Read the model definition and answer for the solid it produces. Units are mm, in the model's axes. Face numbers are marked on the shaded views. A direction names the side the tool comes from. Give positions to 0.01 mm unless a question says otherwise; leave off trailing zeros. Write each loop counter-clockwise with the first axis right and the second up, starting at its lowest first coordinate (ties: lowest second). Pieces come first, ordered by that corner, then holes. Notation, with made-up numbers: (-23, 9.5) -> (-6, 9.5) arc R31 ccw to (-6, 41.5) -> close; hole circle Ø6 at (53, -19). An arc over 180 degrees is marked (long way). Answer as CSV lines item,"result". Start each with the question number.
1. The part is cut by section C-C, the plane y = 531.5. Determine the outline of the cut face in (x, z).
2. Given pin 1 (7.5 mm diameter, centred on x = 5.715, z = 291.592, fed in from -Y); pin 2 (5 mm diameter, centred on x = 15.24, y = 520.7, fed in from -Z); pin 3 (3 mm diameter, centred on y = 525, z = 280, fed in from +X), each flat-ended and moving along its own axis, determine where each tip first touches the part or whether it passes through.
3. Find the intervals of material crossed by line 1 (Z direction, x = 22, y = 526); line 2 (Y direction, x = 15.24, z = 303.95); line 3 (Y direction, x = 28, z = 278.75), in increasing order.
4. The part is cut by section B-B, the plane y = 520.7. Determine the outline of the cut face in (x, z), and give its area (3 significant figures).
5. A tool of negligible diameter and unlimited length cuts with its end or side. For the marked faces 5 and 6, from which of +Z, -Z, +X, -X, +Y, -Y can it reach the whole face along a straight path? Write none if from no direction.
6. For a pull along Z with two mould halves and no side action, classify the marked faces 1, 2, 3 and 4 as pulls with the +Z half, pulls with the -Z half, needs draft (parallel to the pull), parting line crosses it, or undercut.
7. The part is cut by section A-A, the plane x = 15.24. Give the number of separate pieces and of enclosed holes in the cut face, and give its area (3 significant figures).
8. The part is cut by section D-D, the plane x = 24. Determine the outline of the cut face in (y, z) (1 decimal).
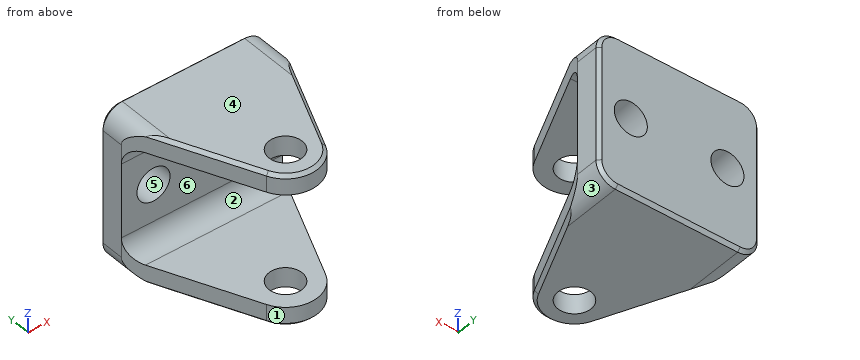
from build123d import *

# Parameters (mm, degrees)
BULK_TRIANGLE_DEPTH      = 14.9225
BULK_TRIANGLE_DEPTH_BACK = 14.9225
U_CUTOUT_DEPTH           = 627.44103
U_CUTOUT_DEPTH_BACK      = 627.44103
F_1_4_CLEARANCE_HOLE1_D  = 6.5278
F_1_4_CLEARANCE_HOLE2_D  = 6.5278
INNER_FILLET_R           = 3.81
TRIANGLE_DEBURR_SIZE     = 0.635
OUTER_FILLET_R           = 3.81
CLAMP_FACE_DEBURR_SIZE   = 0.635


with BuildPart() as part:
    # Sketch1 → Bulk Triangle (new, two sides)
    with BuildSketch(Plane.XY.offset(291.592)) as bulk_triangle_sk:
        with BuildLine():
            Line((9.42744, 518.143313), (-0.635, 541.02))
            Line((-0.635, 541.02), (-0.635, 546.1))
            Line((-0.635, 546.1), (31.115, 546.1))
            Line((31.115, 546.1), (31.115, 541.02))
            Line((31.115, 541.02), (21.05256, 518.143313))
            ThreePointArc((21.05256, 518.143313), (15.24, 514.35), (9.42744, 518.143313))
        make_face()
    extrude(amount=BULK_TRIANGLE_DEPTH)
    extrude(bulk_triangle_sk.sketch, amount=-BULK_TRIANGLE_DEPTH_BACK)

    # Sketch3 → U-Cutout (cut, two sides)
    with BuildSketch(Plane(origin=(15.24, 0, 0), x_dir=(0, -4.31797119152115e-05, -0.9999999990677564), z_dir=(1, 0, 0))) as u_cutout_sk:
        Polygon((-302.727861, 541.006929), (-302.726709, 514.336929), (-280.501709, 514.337888), (-280.502861, 541.007888), align=None)
    extrude(amount=U_CUTOUT_DEPTH, mode=Mode.SUBTRACT)
    extrude(u_cutout_sk.sketch, amount=-U_CUTOUT_DEPTH_BACK, mode=Mode.SUBTRACT)

    # 1/4 Clearance Hole1 (through all)
    with Locations(Plane(origin=(15.24, 520.7, 306.5145), x_dir=(1, 0, 0), z_dir=(0, 0, 1))):
        with Locations((0, 0)):
            Hole(F_1_4_CLEARANCE_HOLE1_D / 2)

    # 1/4 Clearance Hole2 (through all)
    with Locations(Plane(origin=(24.765, 541.02, 291.592), x_dir=(-1, 0, 0), z_dir=(0, -1, 0))):
        with Locations((0, 0), (19.05, 0)):
            Hole(F_1_4_CLEARANCE_HOLE2_D / 2)

    # Inner Fillet
    inner_fillet_edges = [part.edges().sort_by_distance(p)[0] for p in [
        (15.24, 541.02, 280.4795),
        (15.24, 541.02, 302.7045),
    ]]
    fillet(inner_fillet_edges, radius=INNER_FILLET_R)

    # Triangle Deburr
    triangle_deburr_edges = [part.edges().sort_by_distance(p)[0] for p in [
        (15.24, 514.35, 276.6695),
        (4.39622, 529.581656, 276.6695),
        (26.08378, 529.581656, 276.6695),
        (4.39622, 529.581656, 306.5145),
        (15.24, 514.35, 306.5145),
        (26.08378, 529.581656, 306.5145),
    ]]
    chamfer(triangle_deburr_edges, length=TRIANGLE_DEBURR_SIZE)

    # Outer Fillet
    outer_fillet_edges = [part.edges().sort_by_distance(p)[0] for p in [
        (-0.635, 544.348569, 276.6695),
        (31.115, 544.348569, 276.6695),
        (-0.635, 544.348569, 306.5145),
        (31.115, 544.348569, 306.5145),
    ]]
    fillet(outer_fillet_edges, radius=OUTER_FILLET_R)

    # Clamp Face Deburr
    clamp_face_deburr_edges = [part.edges().sort_by_distance(p)[0] for p in [
        (-0.635, 546.1, 291.592),
        (15.24, 546.1, 276.6695),
        (31.115, 546.1, 291.592),
        (15.24, 546.1, 306.5145),
        (29.999077, 546.1, 305.398577),
        (0.480923, 546.1, 305.398577),
        (29.999077, 546.1, 277.785423),
        (0.480923, 546.1, 277.785423),
    ]]
    chamfer(clamp_face_deburr_edges, length=CLAMP_FACE_DEBURR_SIZE)


solid = part.part
Results found:
1,outline,"(3.55, 277.3) -> (4.25, 276.67) -> (26.23, 276.67) -> (26.93, 277.3) -> (26.93, 280.48) -> (3.55, 280.48) -> close; (3.55, 302.7) -> (26.93, 302.7) -> (26.93, 305.88) -> (26.23, 306.51) -> (4.25, 306.51) -> (3.55, 305.88) -> close"
2,pin 1,"stops at y = 541.02"
2,pin 2,"passes through"
2,pin 3,"stops at x = 24.73"
3,line 1,"z = 276.67 to 280.48, 302.7 to 306.51"
3,line 2,"y = 514.35 to 517.44, 523.96 to 546.1"
3,line 3,"y = 533.94 to 546.1"
4,outline,"(8.3, 277.3) -> (9, 276.67) -> (11.98, 276.67) -> (11.98, 280.48) -> (8.3, 280.48) -> close; (8.3, 302.7) -> (11.98, 302.7) -> (11.98, 306.51) -> (9, 306.51) -> (8.3, 305.88) -> close; (18.5, 276.67) -> (21.48, 276.67) -> (22.18, 277.3) -> (22.18, 280.48) -> (18.5, 280.48) -> close; (18.5, 302.7) -> (22.18, 302.7) -> (22.18, 305.88) -> (21.48, 306.51) -> (18.5, 306.51) -> close"
4,area,"55.1 mm²"
5,face 5,"+Y, -Y"
5,face 6,"+X, -X, -Y"
6,face 1,"needs draft"
6,face 2,"undercut"
6,face 3,"pulls with the -Z half"
6,face 4,"pulls with the +Z half"
7,separate pieces,"3"
7,enclosed holes,"0"
7,area,"311 mm²"
8,outline,"(524.8, 277.3) -> (526.4, 276.7) -> (545.5, 276.7) -> (546.1, 277.3) -> (546.1, 288.4) -> (541, 288.4) -> (541, 284.3) arc R3.8 cw to (537.2, 280.5) -> (524.8, 280.5) -> close; (524.8, 302.7) -> (537.2, 302.7) arc R3.8 cw to (541, 298.9) -> (541, 294.8) -> (546.1, 294.8) -> (546.1, 305.9) -> (545.5, 306.5) -> (526.4, 306.5) -> (524.8, 305.9) -> close"
